from build123d import *

# Parameters (mm, degrees)
SKETCH1_W                   = 47
SKETCH1_H                   = 26
BOSS_EXTRUDE1_DEPTH         = 40
CUT_EXTRUDE1_REACH          = 65.071
SKETCH2_W                   = 18
SKETCH2_H                   = 21
FILLET1_R                   = 3
M6_TAPPED_HOLE1_D           = 5
M6_TAPPED_HOLE1_DEPTH       = 15
M6_TAPPED_HOLE1_CSINK_D     = 6.05
M6_TAPPED_HOLE1_CSINK_ANGLE = 90
M6_TAPPED_HOLE1_TIP         = 1.502151548
FILLET2_R                   = 1


with BuildPart() as part:
    # Sketch1 → Boss-Extrude1 (new body)
    with BuildSketch(Plane(origin=(0, 0, 0), x_dir=(1, 0, 0), z_dir=(0, 1, 0))):
        Rectangle(SKETCH1_W, SKETCH1_H)
    extrude(amount=-BOSS_EXTRUDE1_DEPTH)

    # Sketch2 → Cut-Extrude1 (cut, up to next)
    with BuildSketch(Plane(origin=(23.5, 0, 0), x_dir=(0, 0, -1), z_dir=(1, 0, 0)), mode=Mode.PRIVATE) as cut_extrude1_sk1:
        with Locations((-4, -10.5)):
            Rectangle(SKETCH2_W, SKETCH2_H)
    cut_extrude1_tool1 = extrude(cut_extrude1_sk1.sketch, amount=-CUT_EXTRUDE1_REACH, mode=Mode.PRIVATE) & part.part
    add(cut_extrude1_tool1.solids().sort_by_distance((23.5, -10.5, 4))[0], mode=Mode.SUBTRACT)

    # Fillet1
    fillet1_edges = [part.edges().sort_by_distance(p)[0] for p in [
        (0, 0, -5),
        (0, -21, -5),
    ]]
    fillet(fillet1_edges, radius=FILLET1_R)

    # M6 Tapped Hole1
    with Locations(Plane(origin=(0, -40, 0), x_dir=(-1, 0, 0), z_dir=(0, -1, 0))):
        with Locations((-15.5, 0), (15.5, 0)):
            CounterSinkHole(M6_TAPPED_HOLE1_D / 2, M6_TAPPED_HOLE1_CSINK_D / 2, depth=M6_TAPPED_HOLE1_DEPTH, counter_sink_angle=M6_TAPPED_HOLE1_CSINK_ANGLE)
            with Locations((0, 0, -(M6_TAPPED_HOLE1_DEPTH + M6_TAPPED_HOLE1_TIP / 2))):  # 118° drill point
                Cone(0, M6_TAPPED_HOLE1_D / 2, M6_TAPPED_HOLE1_TIP, mode=Mode.SUBTRACT)

    # Fillet2
    fillet2_edges = [part.edges().sort_by_distance(p)[0] for p in [
        (23.5, -30.5, 13),
        (-23.5, -30.5, 13),
        (-23.5, -20, -13),
        (23.5, -20, -13),
    ]]
    fillet(fillet2_edges, radius=FILLET2_R)


solid = part.part
Here's how the part is built. I have some questions about the finished solid (model axes, mm). A direction names the side the tool comes from. Round coordinates to 2 decimals unless told otherwise and drop trailing zeros. Order: outer loops, then holes, each group sorted by start corner. A loop starts at its lowest first (then second) coordinate and runs counter-clockwise, first axis right, second up. Notation, with made-up numbers: (38, 79.5) -> (58, 79.5) arc R34 cw to (58, 114.5) -> close; hole circle Ø8 at (48, -20). An arc over 180 degrees is marked (long way). Return JSON: item names as keys, results as strings.
Q1. If we section it at C-C on y = -16: List the corners of the cut face in (x, z) for me.
Filled sheet:
{"outline": "(-23.5, -12) arc R1 ccw to (-22.5, -13) -> (22.5, -13) arc R1 ccw to (23.5, -12) -> (23.5, -5) -> (-23.5, -5) -> close"}
Q2. If we section it at B-B on x = -8.5: List the corners of the cut face in (y, z) for me.
Filled sheet:
{"outline": "(-40, -13) -> (0, -13) -> (0, -8) arc R3 ccw to (-3, -5) -> (-18, -5) arc R3 cw to (-21, -2) -> (-21, 13) -> (-40, 13) -> close"}
Q3. I need wall thicknesses on line 1 along Z through (x, y) = (15.5, -32.25); line 2 along Y through (x, z) = (9, 6.75); line 3 along Z through (x, y) = (-13.5, -11). Which ranges of each line are inside material? Lowest first, please. Write a range as from..to.
Filled sheet:
{"line 1": "z = -13..-2.5, 2.5..13", "line 2": "y = -40..-21", "line 3": "z = -13..-5"}
Q4. If we mould it in two halves opening along X, with no side actions, what happens to faces 1 (the flat face through (0, -40, 0)), 2 (the cylindrical face through (13, -32, 0)), 3 (the flat face through (23.5, -24, -2))? For each: released by +X, released by -X, zero draft, split by the parting line, or undercut.
Filled sheet:
{"face 1": "zero draft", "face 2": "undercut", "face 3": "released by +X"}
Q5. Which directions (+Z, -Z, +X, -X, +Y, -Y) give clear straight access to the entire face, cutting with the end or side of a thin tool? Please do faces 4 (the flat face through (0, 0, -11)), 5 (the flat face through (0, -21, 6)), 6 (the cylindrical face through (-18, -32, 0)).
Filled sheet:
{"face 4": "+Z, -Z, +X, -X, +Y", "face 5": "+Z, +X, -X, +Y", "face 6": "-Y"}
Q6. If we section it at D-D on z = 4.5: List the corners of the cut face in (x, y) for me.
Filled sheet:
{"outline": "(-23.5, -40) -> (23.5, -40) -> (23.5, -21) -> (-23.5, -21) -> close"}
Q7. For pin 1 Ø7.5 at (x, z) = (6, 2.5) entering from +Y; pin 2 Ø2 at (x, z) = (12, -6) entering from +Y; pin 3 Ø6 at (x, z) = (6, 0) entering from +Y, each with a flat end and sliding along its axis, tell me the tip position at first contact or that it passes through.
Filled sheet:
{"pin 1": "stops at y = -21", "pin 2": "stops at y = -0.17", "pin 3": "stops at y = -20.83"}
Q8. If we section it at A-A on y = -30: List the corners of the cut face in (x, z) for me.
Filled sheet:
{"outline": "(-23.5, -12) arc R1 ccw to (-22.5, -13) -> (22.5, -13) arc R1 ccw to (23.5, -12) -> (23.5, 12) arc R1 ccw to (22.5, 13) -> (-22.5, 13) arc R1 ccw to (-23.5, 12) -> close; hole circle Ø5 at (-15.5, 0); hole circle Ø5 at (15.5, 0)"}
